Check sheet for the modelled part. Datum: model origin and axes. Units: mm. A direction names the side the tool comes from. Give positions to 0.01 mm unless a question says otherwise; leave off trailing zeros. Loops run counter-clockwise (first coordinate to the right, second up) from the corner with the lowest first, then second, coordinate; pieces in that order, holes last. Notation, with made-up numbers: (54.5, 9) -> (88.5, 9) arc R27 ccw to (88.5, 41) -> close; hole circle Ø5 at (53, 2). An arc over 180 degrees is marked (long way). Write each question's results on one line, items separated by ' | '. Start each with the question number.
Item 1: Mould release check, pull along Z, two halves, no side actions. Record for faces 1 (the face through (12, 7, 0)), 2 (the face through (-37, 7, 0)), 3 (the face through (5.158, 6.902, -42.835)): pulls with the +Z half, pulls with the -Z half, needs draft (parallel to the pull), parting line crosses it, or undercut.
Item 2: Gauge pin test, flat ends, axial feed: pin 1 Ø1.5 at (x, y) = (-37.5, 10.5) entering from +Z; pin 2 Ø4 at (x, y) = (3, 6) entering from +Z; pin 3 Ø7.5 at (x, z) = (-4.95, -15) entering from -Y. Record the tip position at first contact, or that the pin passes through.
Item 3: Access from +Z, -Z, +X, -X, +Y, -Y to the whole of each face (thin tool, end or side, straight path). Record for faces 4 (the face through (-4, 3, 12)), 5 (the face through (-2.33, 8.42, -14.17)).
Item 4: Scan lines: line 1 along Z through (x, y) = (0, 10.5); line 2 along Z through (x, y) = (-5.5, 4.25); line 3 along X through (y, z) = (7.5, -35.5). Record each from-to range of solid material in increasing order.
Item 5: Cross-section at B-B on x = 0. Enter the section's corners in (y, z), then the cut area to 3 significant figures.
Item 6: Cross-section at C-C on z = 0. Enter the section's corners in (x, y), then the cut area to 3 significant figures.
Item 7: Cross-section at D-D on x = -42. Enter the section's corners in (y, z), then the cut area to 3 significant figures.
Item 8: Cross-section at A-A on y = 9. Enter the section's corners in (x, z).
Autodesk Inventor part; units mm, degrees
ref_plane "YZ Plane" through (0, 0, 0) normal (1, 0, 0) x (0, 1, 0)
ref_plane "XZ Plane" through (0, 0, 0) normal (0, 1, 0) x (-1, 0, 0)
ref_plane "XY Plane" through (0, 0, 0) normal (0, 0, 1) x (1, 0, 0)
sketch "Sketch1" plane through (0, 0, 0) normal (0, 1, 0) x (-1, 0, 0)
  circle A0 centre (0, 32) radius 5
  circle A1 centre (0, -32) radius 5
  circle A2 centre (42, 0) radius 5
  circle A3 centre (0, -32) radius 12 construction
  circle A4 centre (42, 0) radius 12 construction
  circle A5 centre (0, 32) radius 12 construction
  line L0 (-12, -32) -> (-12, 32)
  line L1 (7.2725, 41.5452) -> (49.2725, 9.5452)
  line L2 (49.2725, -9.5452) -> (7.2725, -41.5452)
  arc A6 (7.2725, 41.5452) -> (-12, 32) centre (0, 32) ccw
  arc A7 (-12, -32) -> (7.2725, -41.5452) centre (0, -32) ccw
  arc A8 (49.2725, -9.5452) -> (49.2725, 9.5452) centre (42, 0) ccw
  point P0 (0, 0)
  dimension "d0" = 10
  dimension "d1" = 64
  dimension "d2" = 32
  dimension "d3" = 24
  dimension "d4" = 42
extrude "Extrusion1" add sketch "Sketch1" along normal blind 14
sketch "Sketch3" plane through (0, 0, 0) normal (0, -1, 0) x (1, 0, 0)
  line L0 (-49.2725, 9.5452) -> (-7.2725, 41.5452) construction
  arc A0 (-49.2725, 9.5452) -> (-49.2725, -9.5452) centre (-42, 0) ccw construction
  line L1 (-7.2725, -41.5452) -> (-49.2725, -9.5452) construction
  arc A1 (-7.2725, -41.5452) -> (12, -32) centre (0, -32) ccw construction
  line L2 (12, 32) -> (12, -32) construction
  arc A2 (12, 32) -> (-7.2725, 41.5452) centre (0, 32) ccw construction
  circle A3 centre (-42, 0) radius 5 construction
  circle A4 centre (0, -32) radius 5 construction
  circle A5 centre (0, 32) radius 5 construction
  line L3 (12, 32) -> (12, -32) construction
  line L4 (12, 0) -> (-42, 0) construction
  line L5 (12, 20) -> (2, 20) construction
  line L6 (2, 20) -> (2, -20) construction
  line L7 (2, -20) -> (12, -20) construction
  line L8 (12, -20) -> (12, 20) construction
  circle A6 centre (-4.95, -15) radius 2.75
  circle A7 centre (-4.95, 15) radius 2.75
  point P0 (0, 0)
  point P1 (7, -20)
  dimension "d7" = 10
  dimension "d8" = 40
  dimension "d9" = 5.5
  dimension "d10" = 5
  dimension "d11" = 6.95
extrude "Extrusion2" cut sketch "Sketch3" against normal through all
sketch "Sketch4" plane through (0, 0, 0) normal (0, -1, 0) x (1, 0, 0)
  circle A0 centre (-4.95, -15) radius 2.75 construction
  circle A1 centre (-4.95, 15) radius 2.75 construction
  line L0 (-49.2725, 9.5452) -> (-7.2725, 41.5452) construction
  arc A2 (-49.2725, 9.5452) -> (-49.2725, -9.5452) centre (-42, 0) ccw construction
  line L1 (-7.2725, -41.5452) -> (-49.2725, -9.5452) construction
  arc A3 (-7.2725, -41.5452) -> (12, -32) centre (0, -32) ccw construction
  line L2 (12, 32) -> (12, -32) construction
  arc A4 (12, 32) -> (-7.2725, 41.5452) centre (0, 32) ccw construction
  circle A5 centre (-42, 0) radius 5 construction
  circle A6 centre (0, -32) radius 5 construction
  circle A7 centre (0, 32) radius 5 construction
  circle A8 centre (-4.95, 15) radius 4.05
  line L3 (-42, 0) -> (0, 0) construction
  circle A9 centre (-4.95, -15) radius 4.05
  dimension "d14" = 8.1
extrude "Extrusion3" cut sketch "Sketch4" against normal blind 3
equation "\"d2\" = 0.5 * d1"
properties part number "base_obj4"
Answer sheet:
1) face 1: needs draft | face 2: undercut | face 3: pulls with the -Z half
2) pin 1: stops at z = 19.09 | pin 2: stops at z = 43.96 | pin 3: stops at y = 3
3) face 4: -Y | face 5: +Y, -Y
4) line 1: z = -44 to -37, -27 to 27, 37 to 44 | line 2: z = -42.67 to -17.69, -12.31 to 12.31, 17.69 to 42.67 | line 3: x = -15.21 to -3.57, 3.57 to 11.48
5) outline: (0, -44) -> (14, -44) -> (14, -37) -> (0, -37) -> close; (0, -27) -> (14, -27) -> (14, 27) -> (0, 27) -> close; (0, 37) -> (14, 37) -> (14, 44) -> (0, 44) -> close | area: 952 mm²
6) outline: (-54, 0) -> (-47, 0) -> (-47, 14) -> (-54, 14) -> close; (-37, 0) -> (12, 0) -> (12, 14) -> (-37, 14) -> close | area: 784 mm²
7) outline: (0, -15.09) -> (14, -15.09) -> (14, -5) -> (0, -5) -> close; (0, 5) -> (14, 5) -> (14, 15.09) -> (0, 15.09) -> close | area: 282 mm²
8) outline: (-49.27, -9.55) -> (-7.27, -41.55) arc R12 ccw to (12, -32) -> (12, 32) arc R12 ccw to (-7.27, 41.55) -> (-49.27, 9.55) arc R12 ccw to start; hole circle Ø10 at (-42, 0); hole circle Ø5.5 at (-4.95, -15); hole circle Ø5.5 at (-4.95, 15); hole circle Ø10 at (0, -32); hole circle Ø10 at (0, 32)
